Geometry check sheet. Reference: the model listing, model coordinates, mm. Face numbers are marked on the shaded views. A direction names the side the tool comes from. Round coordinates to 2 decimals unless told otherwise and drop trailing zeros. Write each loop counter-clockwise with the first axis right and the second up, starting at its lowest first coordinate (ties: lowest second). Pieces come first, ordered by that corner, then holes. Notation, with made-up numbers: (26, -27.5) - (82, -27.5) arc R5 cw to (82, -21.5) - close; hole circle Ø6 at (0, 12.5). An arc over 180 degrees is marked (long way). One line per question, with ' | ' between items. Start each with the question number.
from build123d import *

# Parameters (mm, degrees)
F0_W     = 58.42
F0_H     = 25.4
F1_DEPTH = 25.4
F2_W     = 25.4
F2_H     = 25.4
F3_DEPTH = 25.4
F4_W     = 25.4
F4_H     = 25.4
F5_DEPTH = 25.4


with BuildPart() as f1:
    # F0 (on Right) → F1 (new body)
    with BuildSketch(Plane.YZ):
        with Locations((-33.78506, 17.145792)):
            Rectangle(F0_W, F0_H)
    extrude(amount=F1_DEPTH)

    # F2 (on face) → F3 (join)
    with BuildSketch(Plane(origin=(0, 0, 0), x_dir=(0, -1, 0), z_dir=(-1, 0, 0))):
        with Locations((17.27506, 17.145792)):
            Rectangle(F2_W, F2_H)
    extrude(amount=F3_DEPTH)

    # F4 (on face) → F5 (join)
    with BuildSketch(Plane(origin=(0, 0, 4.445792), x_dir=(1, 0, 0), z_dir=(0, 0, -1))):
        with Locations((-12.7, 17.27506)):
            Rectangle(F4_W, F4_H)
    extrude(amount=F5_DEPTH)


solid = f1.part
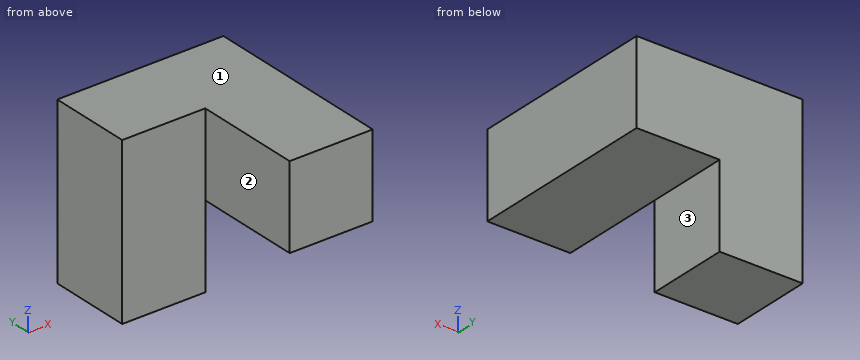
Q1. Section check A-A, the plane y = -17.5. Record the cut outline in (x, z).
Q2. Set-up check for the marked faces 1, 2 and 3: record each of +Z, -Z, +X, -X, +Y, -Y from which the full face is reachable in a straight line by a thin tool's end or side.
Q3. Section check B-B, the plane z = 10. Record the cut outline in (x, y), then the cut area to 3 significant figures.
Q4. Section check C-C, the plane x = 12. Record the cut outline in (y, z), then the cut area to 3 significant figures.
Q5. Go/stop test with flat-tipped pins: P1, Ø20.5, axis at y = -52, z = 21.5, coming from the -X side; P2, Ø7.5, axis at y = -11.5, z = -14, coming from the +X side; P3, Ø12.5, axis at x = 13, y = -39.5, coming from the -Z side. Record where each tip stops, or that it passes through.
Q6. Thickness scan on line 1 (Y direction, x = -13, z = 16); line 2 (X direction, y = -12, z = -19); line 3 (Z direction, x = 2, y = -36). Record the ranges inside material, lowest first.
Q7. Section check D-D, the plane y = -53. Record the cut outline in (x, z).
Result sheet:
1) outline: (-25.4, -20.95) - (0, -20.95) - (0, 4.45) - (25.4, 4.45) - (25.4, 29.85) - (-25.4, 29.85) - close
2) face 1: +Z, +X, -X, +Y, -Y | face 2: +Z, -Z, -X, -Y | face 3: -Z, +X, +Y, -Y
3) outline: (-25.4, -29.98) - (0, -29.98) - (0, -63) - (25.4, -63) - (25.4, -4.58) - (-25.4, -4.58) - close | area: 2,130 mm²
4) outline: (-63, 4.45) - (-4.58, 4.45) - (-4.58, 29.85) - (-63, 29.85) - close | area: 1,480 mm²
5) P1: x = 0 | P2: x = 0 | P3: z = 4.45
6) line 1: -29.98 to -4.58 | line 2: -25.4 to 0 | line 3: 4.45 to 29.85
7) outline: (0, 4.45) - (25.4, 4.45) - (25.4, 29.85) - (0, 29.85) - close
